The listing builds one solid part. Answer for the finished solid, in the listing's coordinates (mm). Face numbers are marked on the shaded views. A direction names the side the tool comes from. Coordinates: 2 decimals unless noted, no trailing zeros. Order: outer loops, then holes, each group sorted by start corner. A loop starts at its lowest first (then second) coordinate and runs counter-clockwise, first axis right, second up. Notation, with made-up numbers: (43.5, 17) - (94.5, 17) arc R22 ccw to (94.5, 55) - close; hole circle Ø3 at (74.25, 46.5). An arc over 180 degrees is marked (long way). Use a Markdown table: item, result. Add a question column.
Item 1: The part is cut by section C-C, the plane y = 2.25. Give the vertices of the cut face in (x, z).
Item 2: For the marked faces 1, 2 and 3, determine the directions among +Z, -Z, +X, -X, +Y, -Y from which every point of the face is accessible in a straight line to the end or side of a thin tool.
Item 3: Find the intervals of material crossed by line 1 along X through (y, z) = (6, 0); line 2 along Y through (x, z) = (-2.5, -3.25); line 3 along Y through (x, z) = (-0.5, -1), in increasing order.
Item 4: The part is cut by section B-B, the plane z = 0. Give the vertices of the cut face in (x, y), then the cut area to 3 significant figures.
Item 5: Flat-ended cylindrical pins translate along their axes: P1, Ø1.4, axis at x = 0, z = 0, coming from the -Y side; P2, Ø4, axis at x = -1.5, y = 22, coming from the +Z side. Find the tip coordinate at first contact, or state that the pin passes through.
Item 6: The mould has two halves that part along X. Classify the marked faces 4, 5 and 6: released by +X, released by -X, zero draft, split by the parting line, or undercut.
Item 7: The part is cut by section D-D, the plane y = 12.25. Give the vertices of the cut face in (x, z), then the cut area to 3 significant figures.
Item 8: The part is cut by section A-A, the plane x = 0. Give the vertices of the cut face in (y, z), then the cut area to 3 significant figures.
from build123d import *

# Parameters (mm, degrees)
SKETCH1_R           = 2.65
BOSS_EXTRUDE1_DEPTH = 15
SKETCH2_R           = 1.15
CUT_EXTRUDE1_DEPTH  = 12
SKETCH3_R           = 4.25
BOSS_EXTRUDE2_DEPTH = 3.7
SKETCH4_R           = 2.9
BOSS_EXTRUDE3_DEPTH = 6
FILLET2_R           = 0.5


with BuildPart() as part:
    # Sketch1 → Boss-Extrude1 (new body)
    with BuildSketch(Plane(origin=(0, 0, 0), x_dir=(1, 0, 0), z_dir=(0, 1, 0))):
        with Locations(Location((0, 0, 0), (0, 0, 270))):
            Circle(SKETCH1_R)
    extrude(amount=BOSS_EXTRUDE1_DEPTH)

    # Sketch2 → Cut-Extrude1 (cut)
    with BuildSketch(Plane.XZ):
        with Locations(Location((0, 0, 0), (0, 0, 270))):
            Circle(SKETCH2_R)
    extrude(amount=-CUT_EXTRUDE1_DEPTH, mode=Mode.SUBTRACT)

    # Sketch3 → Boss-Extrude2 (add)
    with BuildSketch(Plane(origin=(0, 15, 0), x_dir=(1, 0, 0), z_dir=(0, 1, 0))):
        with Locations(Location((0, 0, 0), (0, 0, 270))):
            Circle(SKETCH3_R)
    extrude(amount=BOSS_EXTRUDE2_DEPTH)

    # Sketch4 → Boss-Extrude3 (add)
    with BuildSketch(Plane(origin=(0, 18.7, 0), x_dir=(1, 0, 0), z_dir=(0, 1, 0))):
        with Locations(Location((0, 0, 0), (0, 0, 270))):
            Circle(SKETCH4_R)
    extrude(amount=BOSS_EXTRUDE3_DEPTH)

    # Fillet2
    fillet2_edges = [part.edges().sort_by_distance(p)[0] for p in [
        (0, 24.7, -2.9),
    ]]
    fillet(fillet2_edges, radius=FILLET2_R)


solid = part.part
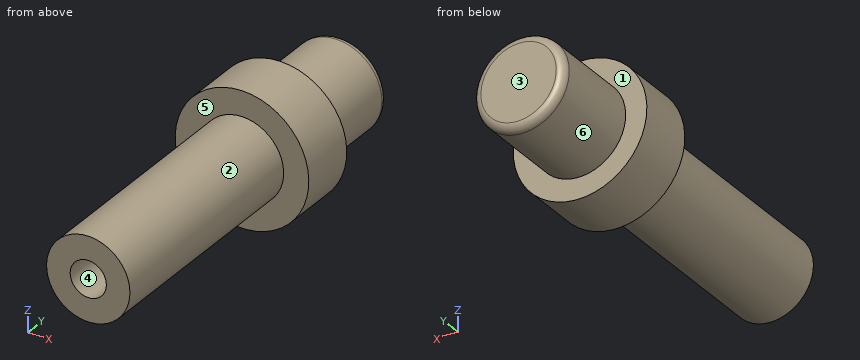
Solution:
| question | item | result |
|---|---|---|
| 1 | outline | circle Ø5.3 at (0, 0); hole circle Ø2.3 at (0, 0) |
| 2 | face 1 | +Y |
| 2 | face 2 | -Y |
| 2 | face 3 | +Z, -Z, +X, -X, +Y |
| 3 | line 1 | x = -2.65 to -1.15, 1.15 to 2.65 |
| 3 | line 2 | y = 15 to 18.7 |
| 3 | line 3 | y = 12 to 24.7 |
| 4 | outline | (-4.25, 15) - (-2.65, 15) - (-2.65, 0) - (-1.15, 0) - (-1.15, 12) - (1.15, 12) - (1.15, 0) - (2.65, 0) - (2.65, 15) - (4.25, 15) - (4.25, 18.7) - (2.9, 18.7) - (2.9, 24.2) arc R0.5 ccw to (2.4, 24.7) - (-2.4, 24.7) arc R0.5 ccw to (-2.9, 24.2) - (-2.9, 18.7) - (-4.25, 18.7) - close |
| 4 | area | 118 mm2 |
| 5 | P1 | stops at y = 12 |
| 5 | P2 | stops at z = 2.9 |
| 6 | face 4 | undercut |
| 6 | face 5 | zero draft |
| 6 | face 6 | split by the parting line |
| 7 | outline | circle Ø5.3 at (0, 0) |
| 7 | area | 22.1 mm2 |
| 8 | outline | (0, -2.65) - (15, -2.65) - (15, -4.25) - (18.7, -4.25) - (18.7, -2.9) - (24.2, -2.9) arc R0.5 ccw to (24.7, -2.4) - (24.7, 2.4) arc R0.5 ccw to (24.2, 2.9) - (18.7, 2.9) - (18.7, 4.25) - (15, 4.25) - (15, 2.65) - (0, 2.65) - (0, 1.15) - (12, 1.15) - (12, -1.15) - (0, -1.15) - close |
| 8 | area | 118 mm2 |
